```python
from build123d import *

# Parameters (mm, degrees)
EXTRUDE_1_DEPTH = 0.5
FILLET_1_R      = 1
EXTRUDE_3_DEPTH = 0.5


with BuildPart() as part:
    # 草图1 → 凸台-拉伸1 (new body)
    with BuildSketch(Plane.XY):
        Polygon((0, 11.32), (-9.803407571, 5.66), (-9.803407571, -5.66), (0, -11.32), (9.803407571, -5.66), (9.803407571, 5.66), align=None)
    extrude(amount=EXTRUDE_1_DEPTH)

    # 圆角1
    fillet_1_edges = [part.edges().sort_by_distance(p)[0] for p in [
        (9.803407571, 5.66, 0.25),
        (9.803407571, -5.66, 0.25),
        (0, -11.32, 0.25),
        (-9.803407571, -5.66, 0.25),
        (-9.803407571, 5.66, 0.25),
        (0, 11.32, 0.25),
    ]]
    fillet(fillet_1_edges, radius=FILLET_1_R)

    # 草图3 → 凸台-拉伸3 (add)
    with BuildSketch(Plane.XY):
        with BuildLine():
            ThreePointArc((-0.705543929, 4.595579399), (-2.307952893, 3.904221506), (-3.711787683, 2.867429289))
            Line((-3.711787683, 2.867429289), (-6.661562741, 4.026250683))
            Line((-6.661562741, 4.026250683), (-6.661562741, 6.935405958))
            Line((-6.661562741, 6.935405958), (-0.705543929, 4.595579399))
        make_face()
        with BuildLine():
            Line((4.934454899, 3.138543991), (4.934454899, 6.0297367))
            Line((4.934454899, 6.0297367), (2.059575955, 4.900778413))
            Line((2.059575955, 4.900778413), (-1.550809491, 3.48298843))
            ThreePointArc((-1.550809491, 3.48298843), (-0.972236897, -5.880889221), (4.037122418, 2.051529715))
            Line((4.037122418, 2.051529715), (1.146295729, 0.94525211))
            ThreePointArc((1.146295729, 0.94525211), (0.382149802, -3.335491783), (-0.835814603, 0.838864453))
            ThreePointArc((-0.835814603, 0.838864453), (-0.56429829, 0.968919842), (-0.277756056, 1.061272752))
            Line((-0.277756056, 1.061272752), (3.527417355, 2.577784143))
            Line((3.527417355, 2.577784143), (4.934454899, 3.138543991))
        make_face()
    extrude(amount=-EXTRUDE_3_DEPTH)


solid = part.part
```
CAD build for the part. Positions are in the model's coordinates, mm. A direction names the side the tool comes from. Round coordinates to 2 decimals unless told otherwise and drop trailing zeros. Write each loop counter-clockwise with the first axis right and the second up, starting at its lowest first coordinate (ties: lowest second). Pieces come first, ordered by that corner, then holes. Notation, with made-up numbers: (-24, 63) - (21, 63) arc R26 cw to (21, 79) - close; hole circle Ø9 at (74.25, -6.5). An arc over 180 degrees is marked (long way). Write item = value, one per line. Start each with the question number.
Q1. Mould opens along X. For faces 1 (the flat face through (2.6, 1.5, -0.2)), 2 (the flat face through (4.84, -8.526, 0.246)), 3 (the cylindrical face through (-2.287, 3.916, -0.246)), 4 (the flat face through (0, 0, 0.5)) say: pulls with the +X half, pulls with the -X half, needs draft (parallel to the pull), parting line crosses it, or undercut.
Q2. Which spindle directions (+Z, -Z, +X, -X, +Y, -Y) get a long thin tool onto all of the face, cutting with end or side? Do faces 5 (the flat face through (4.963, 8.454, 0.246)), 6 (the cylindrical face through (-1.14, -5.835, -0.246)), 7 (the flat face through (0.18, 1.42, -0.5)), 8 (the flat face through (-5.17, 3.44, -0.25)), 9 (the flat face through (-3.725, 5.782, -0.246)). Say none if no direction does.
Q3. Band-saw the part on C-C (x = 1.5). Give the cut face in (y, z), then the cut area to 3 significant figures.
Q4. Band-saw the part on A-A (z = 0.15). Give the cut face in (x, y).
Q5. Drop a flat-ended pin along its axis: pin 1 (0.6 mm diameter, centred on y = 4.5, z = -0.5, fed in from +X). Give the stop position or say it passes through.
Q6. Probe L1, parallel to X at y = -0.75, z = -0.15; L2, parallel to X at y = 0, z = -0.1; L3, parallel to Y at x = 4.75, z = -0.3. List the from-to ranges inside material, lowest first. Write a range as from..to.
Q7. Band-saw the part on B-B (y = -0.25). Give the cut face in (x, z), then the cut area to 3 significant figures.
Q8. Band-saw the part on D-D (y = -4). Give the cut face in (x, z).
Answers below:
q1.face_1 = undercut
q1.face_2 = pulls with the +X half
q1.face_3 = undercut
q1.face_4 = needs draft
q2.face_5 = +Z, -Z, +X, +Y
q2.face_6 = -Z
q2.face_7 = -Z, +X, -X, +Y, -Y
q2.face_8 = -Z, -X
q2.face_9 = -Z, +Y
q3.outline = (-10.45, 0) - (-5.87, 0) - (-5.87, -0.5) - (-2.96, -0.5) - (-2.96, 0) - (0.75, 0) - (0.75, -0.5) - (1.08, -0.5) - (1.08, 0) - (1.77, 0) - (1.77, -0.5) - (4.68, -0.5) - (4.68, 0) - (10.45, 0) - (10.45, 0.5) - (-10.45, 0.5) - close
q3.area = 13.5 mm2
q4.outline = (-9.8, -5.08) arc R1 ccw to (-9.3, -5.95) - (-0.5, -11.03) arc R1 ccw to (0.5, -11.03) - (9.3, -5.95) arc R1 ccw to (9.8, -5.08) - (9.8, 5.08) arc R1 ccw to (9.3, 5.95) - (0.5, 11.03) arc R1 ccw to (-0.5, 11.03) - (-9.3, 5.95) arc R1 ccw to (-9.8, 5.08) - close
q5.pin_1 = 4.93
q6.L1 = -4.67..-1.94, 2.47..5.17
q6.L2 = -4.55..-1.68, 2.2..5.06
q6.L3 = -3.12..0.91, 3.07..5.96
q7.outline = (-9.8, 0) - (-4.6, 0) - (-4.6, -0.5) - (-1.8, -0.5) - (-1.8, 0) - (2.33, 0) - (2.33, -0.5) - (5.11, -0.5) - (5.11, 0) - (9.8, 0) - (9.8, 0.5) - (-9.8, 0.5) - close
q7.area = 12.6 mm2
q8.outline = (-9.8, 0) - (-3.74, 0) - (-3.74, -0.5) - (4.24, -0.5) - (4.24, 0) - (9.8, 0) - (9.8, 0.5) - (-9.8, 0.5) - close
